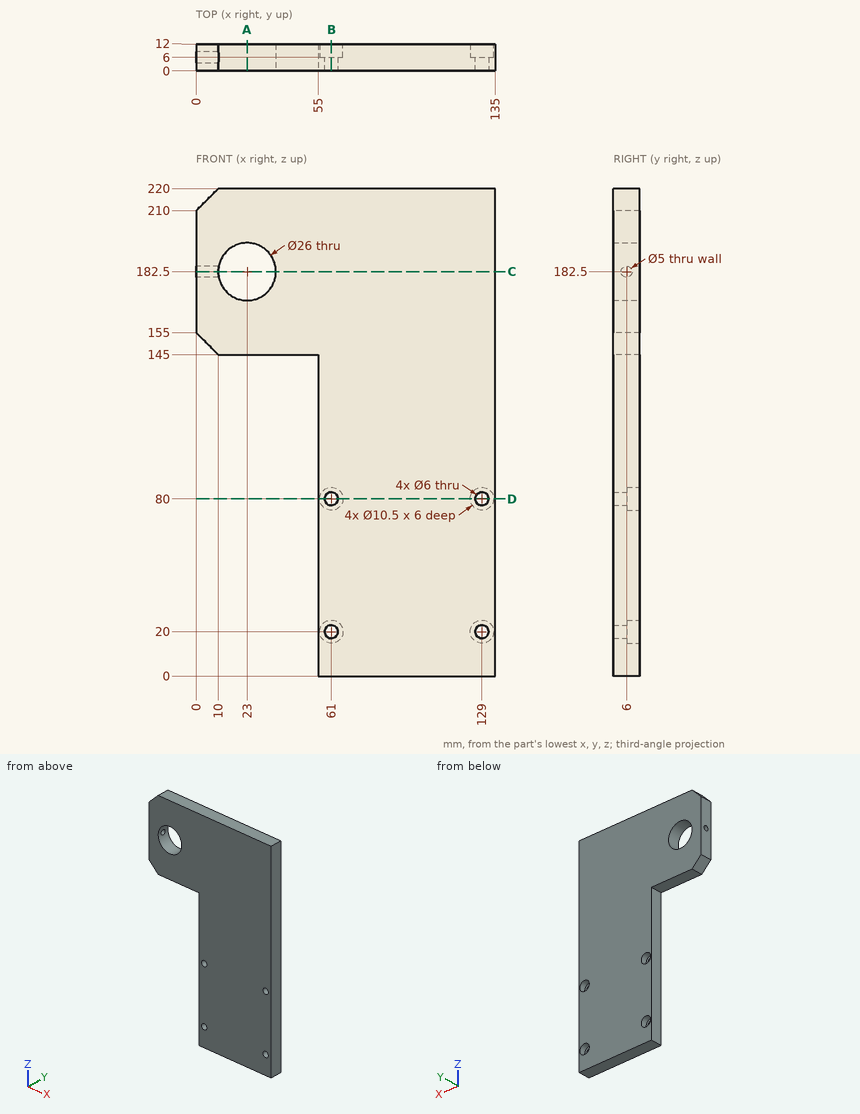
Design review of the part shown in the three views and the two pictorial views. Dimensions are in mm from the part's minimum x, y and z. Give positions to 0.01 mm unless a question says otherwise; leave off trailing zeros. Write each loop counter-clockwise with the first axis right and the second up, starting at its lowest first coordinate (ties: lowest second). Pieces come first, ordered by that corner, then holes.
(1) Wall thickness on line 1 along X through (y, z) = (2.05, 20); line 2 along Z through (x, y) = (129, 1.8); line 3 along Z through (x, y) = (61, 7.65): over which ranges is each line inside the solid? List them lowest first.
Checked values:
line 1: x = 55 to 58, 64 to 126, 132 to 135
line 2: z = 0 to 17, 23 to 77, 83 to 220
line 3: z = 0 to 14.75, 25.25 to 74.75, 85.25 to 220
(2) Add section B-B (x = 61). Give the boundary of the cut face in (y, z).
Checked values:
outline: (0, 0) - (12, 0) - (12, 14.75) - (6, 14.75) - (6, 17) - (0, 17) - close; (0, 23) - (6, 23) - (6, 25.25) - (12, 25.25) - (12, 74.75) - (6, 74.75) - (6, 77) - (0, 77) - close; (0, 83) - (6, 83) - (6, 85.25) - (12, 85.25) - (12, 220) - (0, 220) - close
(3) Add section C-C (z = 182.5). Give the boundary of the cut face in (x, y).
Checked values:
outline: (0, 0) - (10, 0) - (10, 3.5) - (0, 3.5) - close; (0, 8.5) - (10, 8.5) - (10, 12) - (0, 12) - close; (36, 0) - (135, 0) - (135, 12) - (36, 12) - close
(4) Add section D-D (z = 80). Give the boundary of the cut face in (x, y), and give its area (3 significant figures).
Checked values:
outline: (55, 0) - (58, 0) - (58, 6) - (55.75, 6) - (55.75, 12) - (55, 12) - close; (64, 0) - (126, 0) - (126, 6) - (123.75, 6) - (123.75, 12) - (66.25, 12) - (66.25, 6) - (64, 6) - close; (132, 0) - (135, 0) - (135, 12) - (134.25, 12) - (134.25, 6) - (132, 6) - close
area: 762 mm2
(5) Add section A-A (x = 23). Give the boundary of the cut face in (y, z), and give its area (3 significant figures).
Checked values:
outline: (0, 145) - (12, 145) - (12, 169.5) - (0, 169.5) - close; (0, 195.5) - (12, 195.5) - (12, 220) - (0, 220) - close
area: 588 mm2
(6) Clearance check with flat-ended pins moving along their axes: pin 1 Ø1.5 at (y, z) = (8.5, 55) entering from -X; pin 2 Ø5 at (x, z) = (128.5, 79) entering from +Y. State where each tip first meets the part, or that it passes through.
Checked values:
pin 1: stops at x = 55
pin 2: stops at y = 6
